Autodesk Inventor part; units mm, degrees
ref_plane "YZ Plane" through (0, 0, 0) normal (1, 0, 0) x (0, 1, 0)
ref_plane "XZ Plane" through (0, 0, 0) normal (0, 1, 0) x (-1, 0, 0)
ref_plane "XY Plane" through (0, 0, 0) normal (0, 0, 1) x (1, 0, 0)
sketch "Sketch1" plane through (0, 0, 0) normal (0, 0, 1) x (1, 0, 0)
  line L0 (0.3684, -3.4604) -> (14.1917, -1.9888)
  arc A0 (0.3684, 3.4604) -> (0.3684, -3.4604) centre (0, 0) ccw
  line L1 (0.3684, 3.4604) -> (14.1917, 1.9888)
  arc A1 (14.1917, -1.9888) -> (14.1917, 1.9888) centre (13.98, 0) ccw
  line L2 (4.5, -14.3091) -> (27.25, -7.1545)
  line L3 (4.5, 14.3091) -> (27.25, 7.1545)
  arc A2 (27.25, -7.1545) -> (27.25, 7.1545) centre (25, 0) ccw
  arc A3 (4.5, 14.3091) -> (4.5, -14.3091) centre (0, 0) ccw
  dimension "d13" = 3.48
  dimension "d14" = 2
  dimension "d15" = 19.46
  dimension "d17" = 15
  dimension "d18" = 7.5
  dimension "d19" = 25
extrude "Extrusion2" add sketch "Sketch1" along normal blind 3.3
equation "\"d17\" = radio_muslo"
equation "\"d18\" = 0.5 * radio_muslo"
properties part number "Pata - Soporte Antebrazo"
Work out the finished part from the listing and answer in its coordinate system (mm). A direction names the side the tool comes from. Give positions to 0.01 mm unless a question says otherwise; leave off trailing zeros. Loops run counter-clockwise (first coordinate to the right, second up) from the corner with the lowest first, then second, coordinate; pieces in that order, holes last. Notation, with made-up numbers: (70.25, 87.5) -> (123.25, 87.5) arc R26 ccw to (123.25, 125.5) -> close; hole circle Ø10 at (1, 82.25). An arc over 180 degrees is marked (long way). Use a Markdown table: item, result. Add a question column.
1. Section C-C on x = 3 is taken. Determine the outline of the cut face in (y, z), and give its area (3 significant figures).
2. Section D-D on y = -13 is taken. Determine the outline of the cut face in (x, z).
3. Section A-A on y = 0 is taken. Determine the outline of the cut face in (x, z).
4. For faces 1 (the flat face through (7.183, 2.735, 1.627)), 2 (the cylindrical face through (32.5, 0.1, 1.6)), determine the directions among +Z, -Z, +X, -X, +Y, -Y from which every point of the face is accessible in a straight line to the end or side of a thin tool.
5. A flat-ended cylindrical pin translates along its axis: pin 1 Ø2 at (x, y) = (-9, -7) entering from -Z. Find the tip coordinate at first contact, or state that the pin passes through.
6. Determine the mould class of faces 3 (the flat face through (15.72, -10.78, 1.63)), 4 (the flat face through (8, 4, 3.3)), 5 (the cylindrical face through (15.98, 0.04, 1.63)), 6 (the cylindrical face through (-15, 0, 2)) for opening direction X: released by +X, released by -X, zero draft, split by the parting line, or undercut.
7. Find the intervals of material crossed by probe 1 along Y at (x, z) = (0, 1.55); probe 2 along Y at (x, z) = (-2, 1.45); probe 3 along Y at (x, z) = (30, 1.75), in increasing order.
8. Section B-B on z = 1.2 is taken. Determine the outline of the cut face in (x, y).
Results below:
| question | item | result |
|---|---|---|
| 1 | outline | (-14.7, 0) -> (-3.18, 0) -> (-3.18, 3.3) -> (-14.7, 3.3) -> close; (3.18, 0) -> (14.7, 0) -> (14.7, 3.3) -> (3.18, 3.3) -> close |
| 1 | area | 76.0 mm^2 |
| 2 | outline | (-7.48, 0) -> (8.66, 0) -> (8.66, 3.3) -> (-7.48, 3.3) -> close |
| 3 | outline | (-15, 0) -> (-3.48, 0) -> (-3.48, 3.3) -> (-15, 3.3) -> close; (15.98, 0) -> (32.5, 0) -> (32.5, 3.3) -> (15.98, 3.3) -> close |
| 4 | face 1 | +Z, -Z |
| 4 | face 2 | +Z, -Z, +X |
| 5 | pin 1 | stops at z = 0 |
| 6 | face 3 | released by +X |
| 6 | face 4 | zero draft |
| 6 | face 5 | undercut |
| 6 | face 6 | split by the parting line |
| 7 | probe 1 | y = -15 to -3.48, 3.48 to 15 |
| 7 | probe 2 | y = -14.87 to -2.85, 2.85 to 14.87 |
| 7 | probe 3 | y = -5.59 to 5.59 |
| 8 | outline | (4.5, -14.31) -> (27.25, -7.15) arc R7.5 ccw to (27.25, 7.15) -> (4.5, 14.31) arc R15 ccw (long way) to start; hole (0.37, -3.46) -> (14.19, -1.99) arc R2 ccw to (14.19, 1.99) -> (0.37, 3.46) arc R3.48 ccw (long way) to start |
